Geometry check sheet. Reference: the model listing, model coordinates, mm. A direction names the side the tool comes from. Coordinates: 2 decimals unless noted, no trailing zeros. Write each loop counter-clockwise with the first axis right and the second up, starting at its lowest first coordinate (ties: lowest second). Pieces come first, ordered by that corner, then holes.
from build123d import *

# Parameters (mm, degrees)
SKETCH1_R           = 2
BOSS_EXTRUDE1_DEPTH = 10
SKETCH2_W           = 70
SKETCH2_H           = 20
BOSS_EXTRUDE2_DEPTH = 70
CUT_EXTRUDE1_DEPTH  = 20
SKETCH4_R           = 25.5
CUT_EXTRUDE2_DEPTH  = 10
SKETCH5_R           = 15.5
CUT_EXTRUDE3_DEPTH  = 4
SKETCH6_R           = 2.5
CUT_EXTRUDE4_DEPTH  = 10
SKETCH7_R           = 12.5
CUT_EXTRUDE5_DEPTH  = 6
SKETCH8_W           = 20
SKETCH8_H           = 20
CUT_EXTRUDE6_DEPTH  = 15


with BuildPart() as part:
    # Sketch1 → Boss-Extrude1 (new body)
    with BuildSketch(Plane(origin=(0, 0, 0), x_dir=(1, 0, 0), z_dir=(0, 1, 0))):
        Polygon((-35, -40), (-20, -40), (-20, -70), (20, -70), (20, -40), (35, -40), (60, -40), (60, 39), (-60, 39), (-60, -40), align=None)
        with Locations((49.796460718, 28.75)):
            Circle(SKETCH1_R, mode=Mode.SUBTRACT)
        with Locations((49.796460718, -28.75)):
            Circle(SKETCH1_R, mode=Mode.SUBTRACT)
        with Locations((0, -57.5)):
            Circle(SKETCH1_R, mode=Mode.SUBTRACT)
        with Locations((-49.796460718, -28.75)):
            Circle(SKETCH1_R, mode=Mode.SUBTRACT)
        with Locations((-49.796460718, 28.75)):
            Circle(SKETCH1_R, mode=Mode.SUBTRACT)
    extrude(amount=BOSS_EXTRUDE1_DEPTH)

    # Sketch2 → Boss-Extrude2 (add)
    with BuildSketch(Plane(origin=(0, 10, 0), x_dir=(1, 0, 0), z_dir=(0, 1, 0))):
        with Locations((0, 9)):
            Rectangle(SKETCH2_W, SKETCH2_H)
    extrude(amount=BOSS_EXTRUDE2_DEPTH)

    # Sketch3 → Cut-Extrude1 (cut)
    with BuildSketch(Plane(origin=(0, 0, -19), x_dir=(-1, 0, 0), z_dir=(0, 0, -1))):
        with BuildLine():
            ThreePointArc((-35, 45), (-24.748737331, 69.748737352), (3e-08, 80))
            Line((3e-08, 80), (-35, 80))
            Line((-35, 80), (-35, 45))
        make_face()
        with BuildLine():
            Line((35, 45), (35, 80))
            Line((35, 80), (3e-08, 80))
            ThreePointArc((3e-08, 80), (24.748737352, 69.748737331), (35, 45))
        make_face()
    extrude(amount=-CUT_EXTRUDE1_DEPTH, mode=Mode.SUBTRACT)

    # Sketch4 → Cut-Extrude2 (cut)
    with BuildSketch(Plane.XY.offset(1)):
        with Locations((0, 45)):
            Circle(SKETCH4_R)
    extrude(amount=-CUT_EXTRUDE2_DEPTH, mode=Mode.SUBTRACT)

    # Sketch5 → Cut-Extrude3 (cut)
    with BuildSketch(Plane.XY.offset(-9)):
        with Locations((0, 45)):
            Circle(SKETCH5_R)
    extrude(amount=-CUT_EXTRUDE3_DEPTH, mode=Mode.SUBTRACT)

    # Sketch6 → Cut-Extrude4 (cut)
    with BuildSketch(Plane.XY.offset(-9)):
        with Locations((14.142135624, 59.142135624)):
            Circle(SKETCH6_R)
        with Locations((14.142135624, 30.857864376)):
            Circle(SKETCH6_R)
        with Locations((-14.142135624, 30.857864376)):
            Circle(SKETCH6_R)
        with Locations((-14.142135624, 59.142135624)):
            Circle(SKETCH6_R)
    extrude(amount=-CUT_EXTRUDE4_DEPTH, mode=Mode.SUBTRACT)

    # Sketch7 → Cut-Extrude5 (cut)
    with BuildSketch(Plane.XY.offset(-13)):
        with Locations((0, 45)):
            Circle(SKETCH7_R)
    extrude(amount=-CUT_EXTRUDE5_DEPTH, mode=Mode.SUBTRACT)

    # Sketch8 → Cut-Extrude6 (cut)
    with BuildSketch(Plane.XZ):
        Rectangle(SKETCH8_W, SKETCH8_H)
    extrude(amount=-CUT_EXTRUDE6_DEPTH, mode=Mode.SUBTRACT)


solid = part.part
1. Gauge pin test, flat ends, axial feed: pin 1 Ø3 at (x, y) = (-21.5, 66.5) entering from +Z; pin 2 Ø6.5 at (x, z) = (49.8, -28.75) entering from +Y; pin 3 Ø8 at (x, y) = (-14.14, 59.14) entering from -Z. Record the tip position at first contact, or that the pin passes through.
Computed values:
pin 1: stops at z = 1
pin 2: stops at y = 10
pin 3: stops at z = -19
2. Sectioned sample at B-B, the plane z = 57.5. Record the boundary of the cut face in (x, y).
Computed values:
outline: (-20, 0) - (-2, 0) - (-2, 10) - (-20, 10) - close; (2, 0) - (20, 0) - (20, 10) - (2, 10) - close
3. Access from +Z, -Z, +X, -X, +Y, -Y to the whole of each face (thin tool, end or side, straight path). Record for faces 1 (the flat face through (-10, 6, 0)), 2 (the cylindrical face through (-2.018, 60.368, -10.972)), 3 (the flat face through (20, 5, 55)), 4 (the flat face through (-40, 5, 40)), 5 (the flat face through (-35, 27, -9)).
Computed values:
face 1: -Y
face 2: +Z
face 3: +Z, +X, +Y, -Y
face 4: +Z, -X, +Y, -Y
face 5: +Z, -Z, -X, +Y
4. Sectioned sample at A-A, the plane z = -28.75. Record the boundary of the cut face in (x, y).
Computed values:
outline: (-60, 0) - (-51.8, 0) - (-51.8, 10) - (-60, 10) - close; (-47.8, 0) - (47.8, 0) - (47.8, 10) - (-47.8, 10) - close; (51.8, 0) - (60, 0) - (60, 10) - (51.8, 10) - close
5. Sectioned sample at D-D, the plane y = 7. Record the boundary of the cut face in (x, z), and give its area (3 significant figures).
Computed values:
outline: (-60, -39) - (60, -39) - (60, 40) - (20, 40) - (20, 70) - (-20, 70) - (-20, 40) - (-60, 40) - close; hole circle Ø4 at (-49.8, -28.75); hole circle Ø4 at (-49.8, 28.75); hole (-10, -10) - (10, -10) - (10, 10) - (-10, 10) - close; hole circle Ø4 at (0, 57.5); hole circle Ø4 at (49.8, -28.75); hole circle Ø4 at (49.8, 28.75)
area: 10,200 mm2
6. Sectioned sample at C-C, the plane y = 41. Record the boundary of the cut face in (x, z), and give its area (3 significant figures).
Computed values:
outline: (-35, -19) - (-11.84, -19) - (-11.84, -13) - (-14.97, -13) - (-14.97, -9) - (-25.18, -9) - (-25.18, 1) - (-35, 1) - close; (11.84, -19) - (35, -19) - (35, 1) - (25.18, 1) - (25.18, -9) - (14.97, -9) - (14.97, -13) - (11.84, -13) - close
area: 634 mm2
7. Draft check along Z on faces 6 (the cylindrical face through (-51.38, 4.93, -27.53)), 7 (the flat face through (40, 5, 40)), 8 (the flat face through (10, 6, 0)), 9 (the cylindrical face through (-2.71, 32.797, -15.958)). Enter one of: released by +Z, released by -Z, zero draft, split by the parting line, or undercut.
Computed values:
face 6: undercut
face 7: released by +Z
face 8: undercut
face 9: zero draft
8. Thickness scan on line 1 along Z through (x, y) = (0, 2.75); line 2 along X through (y, z) = (2.5, -28.75); line 3 along Y through (x, z) = (0, -3). Record the ranges inside material, lowest first.
Computed values:
line 1: z = -39 to -10, 10 to 55.5, 59.5 to 70
line 2: x = -60 to -51.8, -47.8 to 47.8, 51.8 to 60
line 3: y = 15 to 19.5, 70.5 to 80
